Source: three-view drawing plus pictorial views. Frame: mm from the lowest corner of the part. Give positions to 0.01 mm unless a question says otherwise; leave off trailing zeros. Order: outer loops, then holes, each group sorted by start corner. A loop starts at its lowest first (then second) coordinate and runs counter-clockwise, first axis right, second up.
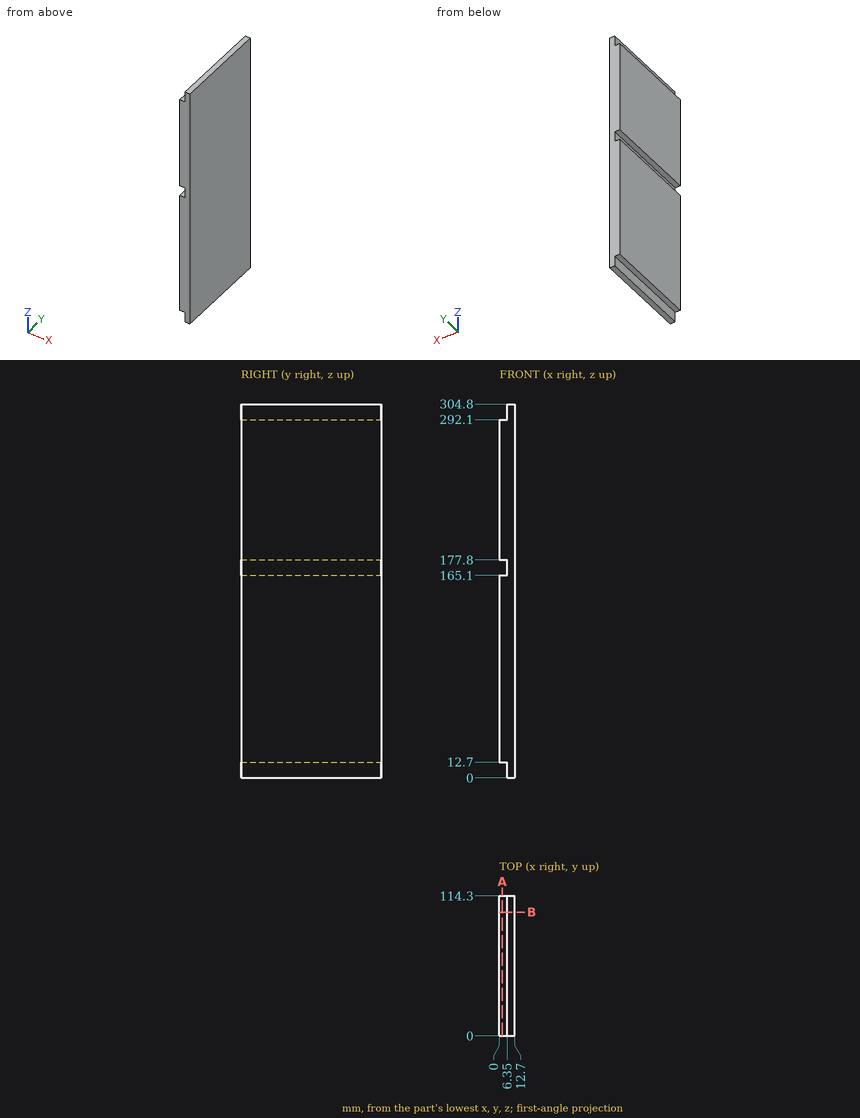
(1) Line query: line 1 along Z through (x, y) = (5.5, 50.5); line 2 along X through (y, z) = (30.5, 167.5). Output: solid intervals per line, ascending.
(2) Section A-A, the plane x = 2.5. Return loops of the section in (y, z), plus the area to 3 significant figures.
(3) Section B-B, the plane y = 101. Return loops of the section in (x, z), plus the area to 3 significant figures.
(4) Pin query (flat end, axial travel): pin 1 Ø1.9 at (x, y) = (2.5, 55.5) entering from +Z; pin 2 Ø10 at (y, z) = (43.5, 298) entering from -X; pin 3 Ø5 at (x, y) = (2.5, 73) entering from -Z. Return the tip coordinate at first contact, or that it passes through.
Checks:
1. line 1: z = 12.7 to 165.1, 177.8 to 292.1
1. line 2: x = 6.35 to 12.7
2. outline: (0, 12.7) - (114.3, 12.7) - (114.3, 165.1) - (0, 165.1) - close; (0, 177.8) - (114.3, 177.8) - (114.3, 292.1) - (0, 292.1) - close
2. area: 30,500 mm2
3. outline: (0, 12.7) - (6.35, 12.7) - (6.35, 0) - (12.7, 0) - (12.7, 304.8) - (6.35, 304.8) - (6.35, 292.1) - (0, 292.1) - (0, 177.8) - (6.35, 177.8) - (6.35, 165.1) - (0, 165.1) - close
3. area: 3,630 mm2
4. pin 1: stops at z = 292.1
4. pin 2: stops at x = 6.35
4. pin 3: stops at z = 12.7
